Geometry check sheet. Reference: the model listing, model coordinates, mm. Face numbers are marked on the shaded views. A direction names the side the tool comes from. Give positions to 0.01 mm unless a question says otherwise; leave off trailing zeros. Loops run counter-clockwise (first coordinate to the right, second up) from the corner with the lowest first, then second, coordinate; pieces in that order, holes last. Notation, with made-up numbers: (77.25, 1) -> (126.25, 1) arc R32 cw to (126.25, 33) -> close; hole circle Ø5 at (18.25, 32). An arc over 180 degrees is marked (long way). Write item = value, one per line.
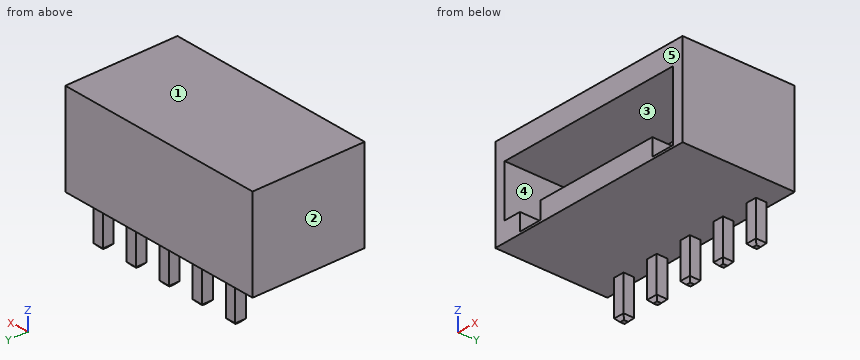
```python
from build123d import *

# Parameters (mm, degrees)
SKETCH_1_W                         = 19.8
SKETCH_1_H                         = 10.5
EXTRUDE_1_DEPTH                    = 8.6
CUT_EXTRUDE_1_DEPTH                = 7
EXTRUDE_START                      = -5
SKETCH_3_W                         = 1
SKETCH_3_H                         = 1
EXTRUDE_2_DEPTH                    = 8.6
CHAMFER_1_SIZE                     = 0.3
PATTERN_LINEAR_1_COUNT             = 5
PATTERN_LINEAR_1_PITCH             = 3.5
CHAMFER_1_OF_PATTERN_LINEAR_1_SIZE = 0.3


with BuildPart() as part:
    # Эскиз1 → Бобышка-Вытянуть1 (new body)
    with BuildSketch(Plane.XY):
        Rectangle(SKETCH_1_W, SKETCH_1_H)
    extrude(amount=EXTRUDE_1_DEPTH)

    # Эскиз2 → Вырез-Вытянуть1 (cut)
    with BuildSketch(Plane.XZ.offset(5.25)):
        Polygon((-8.9, 6.6), (8.9, 6.6), (8.9, 0.2), (6.7, 0.2), (6.7, 1.8), (-5.1, 1.8), (-5.1, 0.2), (-7.3, 0.2), (-7.3, 1.8), (-8.9, 1.8), align=None)
    extrude(amount=-CUT_EXTRUDE_1_DEPTH, mode=Mode.SUBTRACT)

    # Эскиз3 → Бобышка-Вытянуть2 (add)
    with BuildSketch(Plane(origin=(0, 0, 0), x_dir=(-1, 0, 0), z_dir=(0, 0, -1)).offset(EXTRUDE_START)):
        with Locations((7, 4.25)):
            Rectangle(SKETCH_3_W, SKETCH_3_H)
    extrude_2 = extrude(amount=EXTRUDE_2_DEPTH)

    # Фаска1
    chamfer_1_edges = [part.edges().sort_by_distance(p)[0] for p in [
        (-6.5, 4.25, -3.6),
        (-7, 3.75, -3.6),
        (-7.5, 4.25, -3.6),
        (-7, 4.75, -3.6),
    ]]
    chamfer(chamfer_1_edges, length=CHAMFER_1_SIZE)

    # Линейный массив1: Бобышка-Вытянуть2 ×5
    with Locations(*[(i * PATTERN_LINEAR_1_PITCH, 0, 0) for i in range(1, PATTERN_LINEAR_1_COUNT)]):
        add(extrude_2)

    # Фаска1 of Линейный массив1
    chamfer_1_of_pattern_linear_1_edges = [part.edges().sort_by_distance(p)[0] for p in [
        (-3, 4.25, -3.6),
        (-3.5, 3.75, -3.6),
        (-4, 4.25, -3.6),
        (-3.5, 4.75, -3.6),
        (0.5, 4.25, -3.6),
        (0, 3.75, -3.6),
        (-0.5, 4.25, -3.6),
        (0, 4.75, -3.6),
        (4, 4.25, -3.6),
        (3.5, 3.75, -3.6),
        (3, 4.25, -3.6),
        (3.5, 4.75, -3.6),
        (7.5, 4.25, -3.6),
        (7, 3.75, -3.6),
        (6.5, 4.25, -3.6),
        (7, 4.75, -3.6),
    ]]
    chamfer(chamfer_1_of_pattern_linear_1_edges, length=CHAMFER_1_OF_PATTERN_LINEAR_1_SIZE)


solid = part.part
```
Item 1: Thickness scan on L1, parallel to X at y = 4.25, z = -0.5; L2, parallel to X at y = -4, z = 0.75; L3, parallel to Z at x = 0, y = -3.5. Record the ranges inside material, lowest first. Write a range as [from, to].
Answer:
L1 = [-7.5, -6.5], [-4, -3], [-0.5, 0.5], [3, 4], [6.5, 7.5]
L2 = [-9.9, -7.3], [-5.1, 6.7], [8.9, 9.9]
L3 = [0, 1.8], [6.6, 8.6]
Item 2: Gauge pin test, flat ends, axial feed: pin 1 (1.9 mm diameter, centred on x = -1.5, z = 4.5, fed in from -Y); pin 2 (1.1 mm diameter, centred on x = 7, z = -1, fed in from +Y); pin 3 (3 mm diameter, centred on x = 0.5, y = -2.5, fed in from -Z). Record the tip position at first contact, or that the pin passes through.
Answer:
pin_1 = 1.75
pin_2 = 4.75
pin_3 = 0
Item 3: Section check A-A, the plane z = -1. Record the cut outline in (x, y).
Answer:
outline = (-7.5, 3.75) -> (-6.5, 3.75) -> (-6.5, 4.75) -> (-7.5, 4.75) -> close; (-4, 3.75) -> (-3, 3.75) -> (-3, 4.75) -> (-4, 4.75) -> close; (-0.5, 3.75) -> (0.5, 3.75) -> (0.5, 4.75) -> (-0.5, 4.75) -> close; (3, 3.75) -> (4, 3.75) -> (4, 4.75) -> (3, 4.75) -> close; (6.5, 3.75) -> (7.5, 3.75) -> (7.5, 4.75) -> (6.5, 4.75) -> close
Item 4: Draft check along Z on the marked faces 1, 2 and 3. Enter one of: +Z half, -Z half, draft (parallel to the pull), parting line (faces both ways), or undercut.
Answer:
face_1 = +Z half
face_2 = draft
face_3 = undercut
Item 5: Section check B-B, the plane y = -4.5. Record the cut outline in (x, z), plus the area to 3 significant figures.
Answer:
outline = (-9.9, 0) -> (9.9, 0) -> (9.9, 8.6) -> (-9.9, 8.6) -> close; hole (-8.9, 1.8) -> (-7.3, 1.8) -> (-7.3, 0.2) -> (-5.1, 0.2) -> (-5.1, 1.8) -> (6.7, 1.8) -> (6.7, 0.2) -> (8.9, 0.2) -> (8.9, 6.6) -> (-8.9, 6.6) -> close
area = 77.8 mm^2
Item 6: Section check C-C, the plane x = -6.25. Record the cut outline in (y, z), plus the area to 3 significant figures.
Answer:
outline = (-5.25, 0) -> (5.25, 0) -> (5.25, 8.6) -> (-5.25, 8.6) -> (-5.25, 6.6) -> (1.75, 6.6) -> (1.75, 0.2) -> (-5.25, 0.2) -> close
area = 45.5 mm^2
Item 7: Section check D-D, the plane z = 4.25. Record the cut outline in (x, y).
Answer:
outline = (-9.9, -5.25) -> (-8.9, -5.25) -> (-8.9, 1.75) -> (8.9, 1.75) -> (8.9, -5.25) -> (9.9, -5.25) -> (9.9, 5.25) -> (-9.9, 5.25) -> close
Item 8: Tool access check on the marked faces 4 and 5. Record the directions out of +Z, -Z, +X, -X, +Y, -Y that give a thin tool (end or side, any length) a straight path to the whole face; none if there is none.
Answer:
face_4 = -Y
face_5 = +Z, -Z, +X, -X, -Y
